Check sheet for the drawn part. Datum: minimum x, y, z corner. Units: mm. Coordinates: 2 decimals unless noted, no trailing zeros. Loops run counter-clockwise (first coordinate to the right, second up) from the corner with the lowest first, then second, coordinate; pieces in that order, holes last. Notation, with made-up numbers: (83.5, 31) - (114.5, 31) arc R21 cw to (114.5, 61) - close; hole circle Ø6 at (-2, 48). An arc over 180 degrees is marked (long way). Answer as a JSON object with one key per item and string values. Group by question number.
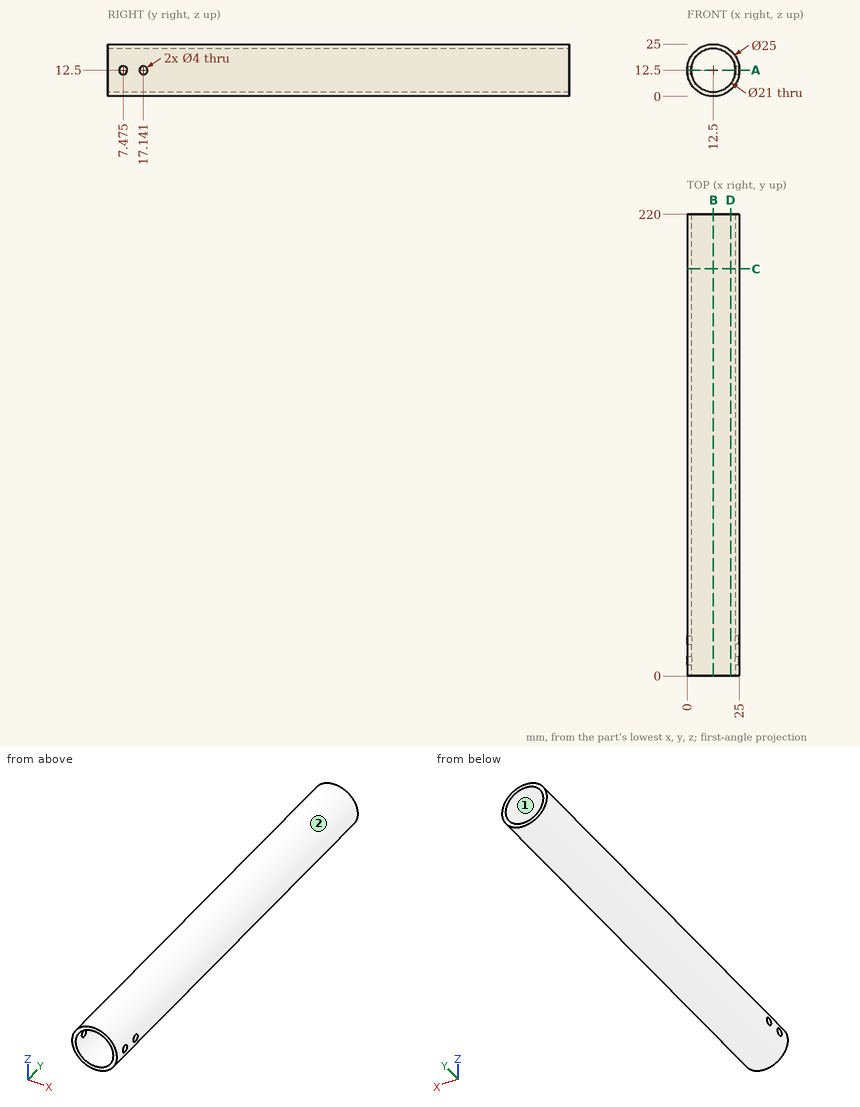
1. Release check for a two-part mould opening along Z. For the marked faces 1 and 2 record: released by +Z, released by -Z, zero draft, split by the parting line, or undercut.
2. Gauge pin test, flat ends, axial feed: pin 1 (5 mm diameter, centred on x = 7.5, z = 21, fed in from -Y); pin 2 (3 mm diameter, centred on x = 9, z = 19, fed in from +Y); pin 3 (2 mm diameter, centred on y = 54, z = 5, fed in from +X); pin 4 (1 mm diameter, centred on y = 44.5, z = 6, fed in from -X). Record the tip position at first contact, or that the pin passes through.
3. Sectioned sample at B-B on x = 12.5. Record the cut outline in (y, z), plus the area to 3 significant figures.
4. Sectioned sample at C-C on y = 194. Record the cut outline in (x, z), plus the area to 4 significant figures.
5. Sectioned sample at D-D on x = 20.75. Record the cut outline in (y, z) (3 decimals).
6. Material ranges on line 1 (Y direction, x = 23.8, z = 12.5) (3 decimals); line 2 (X direction, y = 122, z = 12); line 3 (Z direction, x = 14.25, y = 76), recorded low to high.
7. Sectioned sample at A-A on z = 12.5. Record the cut outline in (x, y) (3 decimals), plus the area to 3 significant figures.
Answers follow:
{
 "1": {"face 1": "undercut", "face 2": "split by the parting line"},
 "2": {"pin 1": "stops at y = 0", "pin 2": "passes through", "pin 3": "stops at x = 23.18", "pin 4": "stops at x = 1.53"},
 "3": {"outline": "(0, 0) - (220, 0) - (220, 2) - (0, 2) - close; (0, 23) - (220, 23) - (220, 25) - (0, 25) - close", "area": "880 mm^2"},
 "4": {"outline": "circle Ø25 at (12.5, 12.5); hole circle Ø21 at (12.5, 12.5)", "area": "144.5 mm^2"},
 "5": {"outline": "(0, 3.109) - (220, 3.109) - (220, 6.005) - (0, 6.005) - close; (0, 18.995) - (220, 18.995) - (220, 21.891) - (0, 21.891) - close"},
 "6": {"line 1": "y = 0 to 5.475, 9.475 to 15.141, 19.141 to 220", "line 2": "x = 0.01 to 2.01, 22.99 to 24.99", "line 3": "z = 0.12 to 2.15, 22.85 to 24.88"},
 "7": {"outline": "(0, 0) - (2, 0) - (2, 5.475) - (0, 5.475) - close; (0, 9.475) - (2, 9.475) - (2, 15.141) - (0, 15.141) - close; (0, 19.141) - (2, 19.141) - (2, 220) - (0, 220) - close; (23, 0) - (25, 0) - (25, 5.475) - (23, 5.475) - close; (23, 9.475) - (25, 9.475) - (25, 15.141) - (23, 15.141) - close; (23, 19.141) - (25, 19.141) - (25, 220) - (23, 220) - close", "area": "848 mm^2"}
}
